Geometry: final body of the model. Coordinates: model frame, mm. A direction names the side the tool comes from. Coordinates: 2 decimals unless noted, no trailing zeros. Order: outer loops, then holes, each group sorted by start corner. A loop starts at its lowest first (then second) coordinate and runs counter-clockwise, first axis right, second up. Notation, with made-up numbers: (-37, 87) -> (-16, 87) arc R28 ccw to (-16, 112) -> close; hole circle Ø10 at (62.5, 45). An arc over 180 degrees is marked (long way). Use one line per item in the form item = value.
```python
from build123d import *

# Parameters (mm, degrees)
SKETCH_1_W          = 20
SKETCH_1_H          = 20
EXTRUDE_1_DEPTH     = 2
SKETCH_2_W          = 20
SKETCH_2_H          = 2
EXTRUDE_2_DEPTH     = 18
SKETCH_3_R          = 1.5
CUT_EXTRUDE_1_DEPTH = 10
SKETCH_4_R          = 1.5
CUT_EXTRUDE_2_DEPTH = 10


with BuildPart() as part:
    # 草图1 → 凸台-拉伸1 (new body)
    with BuildSketch(Plane.XY):
        Rectangle(SKETCH_1_W, SKETCH_1_H)
    extrude(amount=EXTRUDE_1_DEPTH)

    # 草图2 → 凸台-拉伸2 (add)
    with BuildSketch(Plane.XY.offset(2)):
        with Locations((0, -9)):
            Rectangle(SKETCH_2_W, SKETCH_2_H)
    extrude(amount=EXTRUDE_2_DEPTH)

    # 草图3 → 切除-拉伸1 (cut)
    with BuildSketch(Plane.XY.offset(2)):
        with Locations((-5, 0)):
            Circle(SKETCH_3_R)
    extrude(amount=-CUT_EXTRUDE_1_DEPTH, mode=Mode.SUBTRACT)

    # 草图4 → 切除-拉伸2 (cut)
    with BuildSketch(Plane(origin=(0, -8, 0), x_dir=(1, 0, 0), z_dir=(0, 1, 0))):
        with Locations(Location((5, -10, 0), (0, 0, 270))):
            Circle(SKETCH_4_R)
    extrude(amount=-CUT_EXTRUDE_2_DEPTH, mode=Mode.SUBTRACT)


solid = part.part
```
1) Section C-C, the plane z = 10. Output: boundary loops of the cut face in (x, y), and give its area (3 significant figures).
Results found:
outline = (-10, -10) -> (3.5, -10) -> (3.5, -8) -> (-10, -8) -> close; (6.5, -10) -> (10, -10) -> (10, -8) -> (6.5, -8) -> close
area = 34.0 mm2
2) Access query for faces 4 (the flat face through (0, 1, 2)), 5 (the cylindrical face through (5.07, -8.99, 8.5)). Directions: +Z, -Z, +X, -X, +Y, -Y. A direction counts if a zero-diameter tool reaches every point of the face in a straight line with its end or side. Return the directions, or none.
Results found:
face_4 = +Z, +X, -X, +Y
face_5 = +Y, -Y
3) Material intervals for probe 1 along Y at (x, z) = (-5, 0.45); probe 2 along X at (y, z) = (-8.6, 10); probe 3 along Y at (x, z) = (-4, 10.25), sorted ascending. Write a range as from..to.
Results found:
probe_1 = -10..-1.5, 1.5..10
probe_2 = -10..3.5, 6.5..10
probe_3 = -10..-8
4) Contact query for flat-ended pins moving along their axis: P1, Ø8, axis at x = 0, y = -2, coming from the +Z side; P2, Ø1.8, axis at x = -5, y = 0, coming from the +Z side; P3, Ø12, axis at x = -1.5, y = -6, coming from the -Z side; P4, Ø5, axis at x = 5, z = 10, coming from the +Y side. Output: stop coordinate, or through.
Results found:
P1 = 2
P2 = through
P3 = 0
P4 = -8
5) Pull-direction query (X, two-part tool) for faces 1 (the cylindrical face through (-6.2, -0.9, 1)), 2 (the flat face through (10, -8.2, 5.5)), 3 (the flat face through (0, -9, 20)); classes: released by +X, released by -X, zero draft, split by the parting line, or undercut.
Results found:
face_1 = undercut
face_2 = released by +X
face_3 = zero draft
6) Section A-A, the plane x = 5. Output: boundary loops of the cut face in (y, z), and give its area (3 significant figures).
Results found:
outline = (-10, 0) -> (10, 0) -> (10, 2) -> (-8, 2) -> (-8, 8.5) -> (-10, 8.5) -> close; (-10, 11.5) -> (-8, 11.5) -> (-8, 20) -> (-10, 20) -> close
area = 70.0 mm2
7) Section B-B, the plane z = 1.5. Output: boundary loops of the cut face in (x, y), and give its area (3 significant figures).
Results found:
outline = (-10, -10) -> (10, -10) -> (10, 10) -> (-10, 10) -> close; hole circle Ø3 at (-5, 0)
area = 393 mm2
8) Section D-D, the plane x = 2.5. Output: boundary loops of the cut face in (y, z), and give its area (3 significant figures).
Results found:
outline = (-10, 0) -> (10, 0) -> (10, 2) -> (-8, 2) -> (-8, 20) -> (-10, 20) -> close
area = 76.0 mm2
